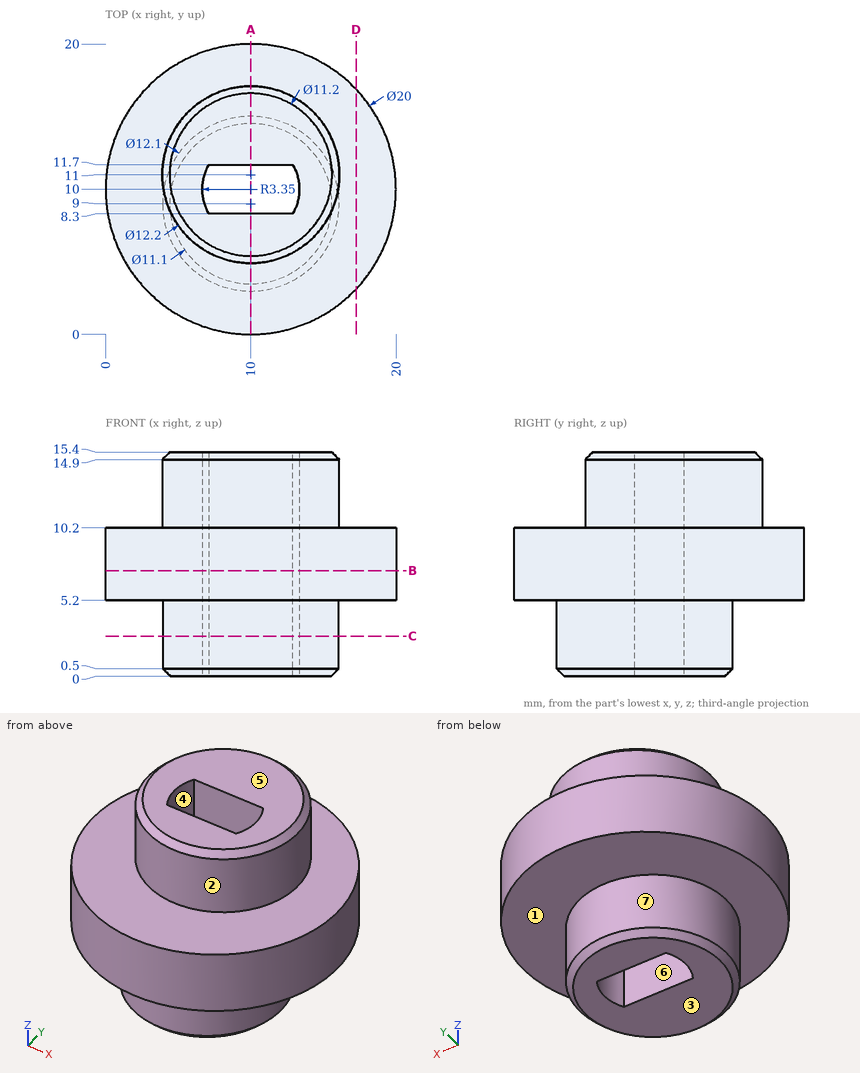
Geometry check sheet. Reference: drawing and pictorial views, mm from the part's lowest x, y, z. A direction names the side the tool comes from. Coordinates: 2 decimals unless noted, no trailing zeros. Order: outer loops, then holes, each group sorted by start corner. A loop starts at its lowest first (then second) coordinate and runs counter-clockwise, first axis right, second up.
Item 1: Section check D-D (x = 17.25). Enter the section's corners in (y, z).
Item 2: Mould release check, pull along Y, two halves, no side actions. Record for the marked faces 5, 6 and 7: released by +Y, released by -Y, zero draft, split by the parting line, or undercut.
Item 3: Depth check by flat-ended pin: pin 1 (2 mm diameter, centred on y = 12.5, z = 12, fed in from +X); pin 2 (1.5 mm diameter, centred on x = 3.5, y = 2.5, fed in from -Z); pin 3 (3 mm diameter, centred on x = 6.5, z = 7, fed in from +Y). Enter the tip coordinate at first touch or a pass-through.
Item 4: Section check A-A (x = 10). Enter the section's corners in (y, z), plus the area to 4 significant figures.
Item 5: Tool access check on the marked faces 1, 2, 3 and 4. Record the directions out of +Z, -Z, +X, -X, +Y, -Y that give a thin tool (end or side, any length) a straight path to the whole face; none if there is none.
Item 6: Section check B-B (z = 7.25). Enter the section's corners in (x, y), plus the area to 3 significant figures.
Item 7: Section check C-C (z = 2.75). Enter the section's corners in (x, y), plus the area to 3 significant figures.
Item 8: Scan lines: line 1 along Z through (x, y) = (12.75, 17); line 2 along X through (y, z) = (10.25, 5.75); line 3 along Y through (x, z) = (13, 9.5). Record each from-to range of solid material in increasing order.
Check sheet entries:
1. outline: (3.11, 5.2) - (16.89, 5.2) - (16.89, 10.2) - (3.11, 10.2) - close
2. face 5: zero draft
2. face 6: undercut
2. face 7: split by the parting line
3. pin 1: stops at x = 16.08
3. pin 2: stops at z = 5.2
3. pin 3: stops at y = 19.8
4. outline: (0, 5.2) - (2.95, 5.2) - (2.95, 0.5) - (3.45, 0) - (8.3, 0) - (8.3, 15.4) - (5.4, 15.4) - (4.9, 14.9) - (4.9, 10.2) - (0, 10.2) - close; (11.7, 0) - (14.55, 0) - (15.05, 0.5) - (15.05, 5.2) - (20, 5.2) - (20, 10.2) - (17.1, 10.2) - (17.1, 14.9) - (16.6, 15.4) - (11.7, 15.4) - close
4. area: 173.5 mm2
5. face 1: -Z
5. face 2: +Z
5. face 3: -Z, +X, -X, +Y, -Y
5. face 4: +Z, -Z
6. outline: circle Ø20 at (10, 10); hole (7.11, 8.3) - (12.89, 8.3) arc R3.35 ccw to (12.89, 11.7) - (7.11, 11.7) arc R3.35 ccw to start
6. area: 292 mm2
7. outline: circle Ø12.1 at (10, 9); hole (7.11, 8.3) - (12.89, 8.3) arc R3.35 ccw to (12.89, 11.7) - (7.11, 11.7) arc R3.35 ccw to start
7. area: 93.2 mm2
8. line 1: z = 5.2 to 10.2
8. line 2: x = 0 to 6.66, 13.34 to 20
8. line 3: y = 0.46 to 8.51, 11.49 to 19.54
